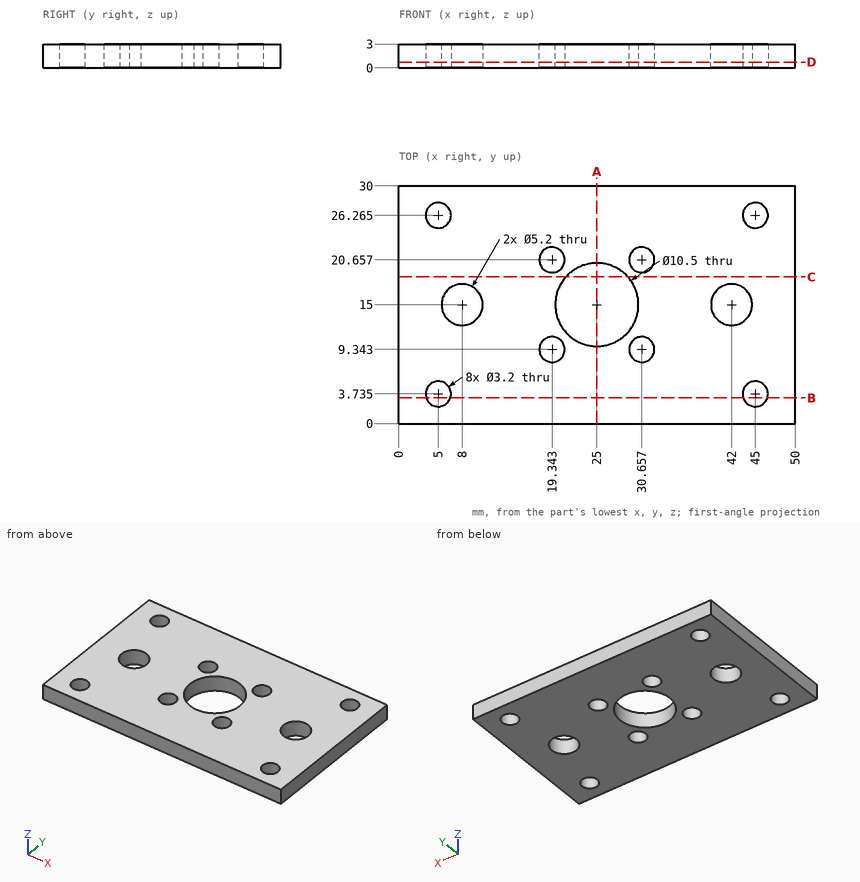
Print and shaded views of the part. All mm, measured from the part's lowest x, y and z. Coordinates: 2 decimals unless noted, no trailing zeros. Order: outer loops, then holes, each group sorted by start corner. A loop starts at its lowest first (then second) coordinate and runs counter-clockwise, first axis right, second up. Notation, with made-up numbers: (24, 47) - (51, 47) arc R24 cw to (51, 85) - close; hole circle Ø7 at (36, 33.25). An arc over 180 degrees is marked (long way). Put each result on its own line as item: value.
1. Saw through at A-A (x = 25). Write the cut outline in (y, z).
Answer sheet:
outline: (0, 0) - (9.75, 0) - (9.75, 3) - (0, 3) - close; (20.25, 0) - (30, 0) - (30, 3) - (20.25, 3) - close
2. Saw through at D-D (z = 0.7). Give the number of separate pieces and of enclosed holes in the cut face, and give its area (3 significant figures).
Answer sheet:
separate pieces: 1
enclosed holes: 11
area: 1,310 mm^2
3. Drop flat-ended pins along their axis: P1, Ø5, axis at x = 5, y = 3.73, coming from the -Z side; P2, Ø1.9, axis at x = 30.66, y = 9.34, coming from the -Z side. Give the stop position or say it passes through.
Answer sheet:
P1: stops at z = 0
P2: passes through
4. Saw through at C-C (y = 18.5). Write the cut outline in (x, z).
Answer sheet:
outline: (0, 0) - (21.09, 0) - (21.09, 3) - (0, 3) - close; (28.91, 0) - (50, 0) - (50, 3) - (28.91, 3) - close
5. Saw through at B-B (y = 3.25). Write the cut outline in (x, z) (1 decimal).
Answer sheet:
outline: (0, 0) - (3.5, 0) - (3.5, 3) - (0, 3) - close; (6.5, 0) - (43.5, 0) - (43.5, 3) - (6.5, 3) - close; (46.5, 0) - (50, 0) - (50, 3) - (46.5, 3) - close
6. Probe line 1 along Y through (x, z) = (5, 1.95) (1 decimal); line 2 along X through (y, z) = (2.75, 2.7); line 3 along X through (y, z) = (3.5, 0.55). List the from-to ranges inside material, lowest first. Write a range as [from, to].
Answer sheet:
line 1: y = [0, 2.1], [5.3, 24.7], [27.9, 30]
line 2: x = [0, 3.74], [6.26, 43.74], [46.26, 50]
line 3: x = [0, 3.42], [6.58, 43.42], [46.58, 50]
